Design review of the part built by this model. Coordinates are the model's own, in mm. Face numbers are marked on the shaded views. Round coordinates to 2 decimals unless told otherwise and drop trailing zeros. Write each loop counter-clockwise with the first axis right and the second up, starting at its lowest first coordinate (ties: lowest second). Pieces come first, ordered by that corner, then holes.
from build123d import *

# Parameters (mm, degrees)
SKETCH1_W                   = 25.4
SKETCH1_H                   = 12.7
EXTRUDE1_DEPTH              = 34.925
CHAMFER1_SIZE               = 10.16
CHAMFER1_SIZE2              = 1.427894881
F_1_4_0_25_DIAMETER_HOLE1_D = 6.35
EXTRUDE2_DEPTH              = 13.7


with BuildPart() as part:
    # Sketch1 → Extrude1 (new body)
    with BuildSketch(Plane.XY):
        Rectangle(SKETCH1_W, SKETCH1_H)
    extrude(amount=EXTRUDE1_DEPTH)

    # Chamfer1
    chamfer1_edges = [part.edges().sort_by_distance(p)[0] for p in [
        (12.7, -6.35, 17.4625),
        (-12.7, -6.35, 17.4625),
    ]]
    chamfer1_side = [part.faces().sort_by_distance(p)[0] for p in [
        (0, -6.35, 17.4625),
    ]]
    chamfer(chamfer1_edges, length=CHAMFER1_SIZE, length2=CHAMFER1_SIZE2, reference=chamfer1_side[0])

    # 1/4 (0.25) Diameter Hole1 (through all)
    with Locations(Plane(origin=(0, 0, 0), x_dir=(-1, 0, 0), z_dir=(0, 0, -1))):
        with Locations((0, -1.27)):
            Hole(F_1_4_0_25_DIAMETER_HOLE1_D / 2)

    # Sketch5 → Extrude2 (cut, through all)
    with BuildSketch(Plane(origin=(0, 6.35, 0), x_dir=(1, 0, 0), z_dir=(0, 1, 0))):
        with BuildLine():
            Line((-11.27125, -11.77925), (-12.7, -11.77925))
            Line((-12.7, -11.77925), (-12.7, -7.01675))
            Line((-12.7, -7.01675), (-11.27125, -7.01675))
            ThreePointArc((-11.27125, -7.01675), (-8.89, -9.398), (-11.27125, -11.77925))
        make_face()
    extrude2 = extrude(amount=-EXTRUDE2_DEPTH, mode=Mode.SUBTRACT)

    # Mirror1: Extrude2 across plane
    add(extrude2.mirror(Plane(origin=(0, 0, 0), x_dir=(0, 0, 1), z_dir=(1, 0, 0))), mode=Mode.SUBTRACT)


solid = part.part
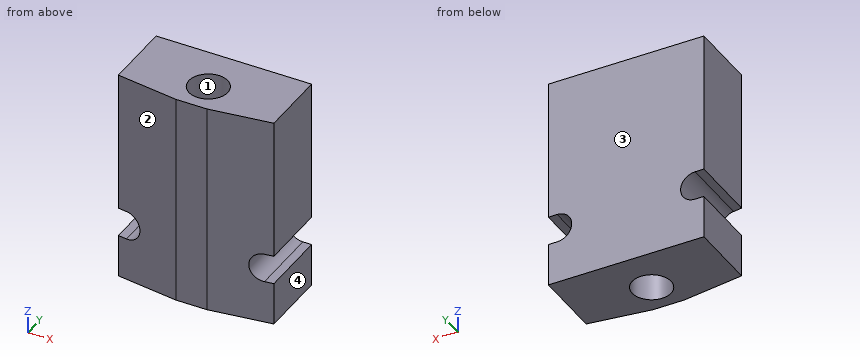
1) The part is to be moulded in two halves that separate along Y. For the marked faces 1, 2, 3 and 4, say which applies: pulls with the +Y half, pulls with the -Y half, needs draft (parallel to the pull), parting line crosses it, or undercut.
2) For line 1 along Y through (x, z) = (0, 13) (3 decimals); line 2 along X through (y, z) = (-1.5, 4); line 3 along X through (y, z) = (-0.75, 8.5), list the stretches that pass through material, from the lowest coordinate up.
3) Add section A-A on y = -1.27. State the section outline as (x, z) points (1 decimal).
4) Add section B-B on x = 0. State the section outline as (y, z) points (3 decimals).
5) Add section D-D on y = 0.75. State the section outline as (x, z) points (1 decimal).
6) Add section C-C on y = 5.5. State the section outline as (x, z) points (1 decimal), and give its area (3 significant figures).
7) For P1, Ø2, axis at x = 2, y = -2, coming from the -Z side, flat-tipped, find the tip position at first contact; note if it passes through.
Computed:
1. face 1: undercut
1. face 2: pulls with the -Y half
1. face 3: pulls with the +Y half
1. face 4: needs draft
2. line 1: y = -6.35 to -4.445, 1.905 to 6.35
2. line 2: x = -12.7 to -3.17, 3.17 to 12.7
2. line 3: x = -9.07 to -3.13, 3.13 to 9.07
3. outline: (-12.7, 0) - (-3.2, 0) - (-3.2, 34.9) - (-12.7, 34.9) - (-12.7, 11.8) - (-11.3, 11.8) arc R2.4 cw to (-11.3, 7) - (-12.7, 7) - close; (3.2, 0) - (12.7, 0) - (12.7, 7) - (11.3, 7) arc R2.4 cw to (11.3, 11.8) - (12.7, 11.8) - (12.7, 34.9) - (3.2, 34.9) - close
4. outline: (-6.35, 0) - (-4.445, 0) - (-4.445, 34.925) - (-6.35, 34.925) - close; (1.905, 0) - (6.35, 0) - (6.35, 34.925) - (1.905, 34.925) - close
5. outline: (-12.7, 0) - (-2.4, 0) - (-2.4, 34.9) - (-12.7, 34.9) - (-12.7, 11.8) - (-11.3, 11.8) arc R2.4 cw to (-11.3, 7) - (-12.7, 7) - close; (2.4, 0) - (12.7, 0) - (12.7, 7) - (11.3, 7) arc R2.4 cw to (11.3, 11.8) - (12.7, 11.8) - (12.7, 34.9) - (2.4, 34.9) - close
6. outline: (-12.7, 0) - (12.7, 0) - (12.7, 7) - (11.3, 7) arc R2.4 cw to (11.3, 11.8) - (12.7, 11.8) - (12.7, 34.9) - (-12.7, 34.9) - (-12.7, 11.8) - (-11.3, 11.8) arc R2.4 cw to (-11.3, 7) - (-12.7, 7) - close
6. area: 856 mm2
7. P1: passes through
